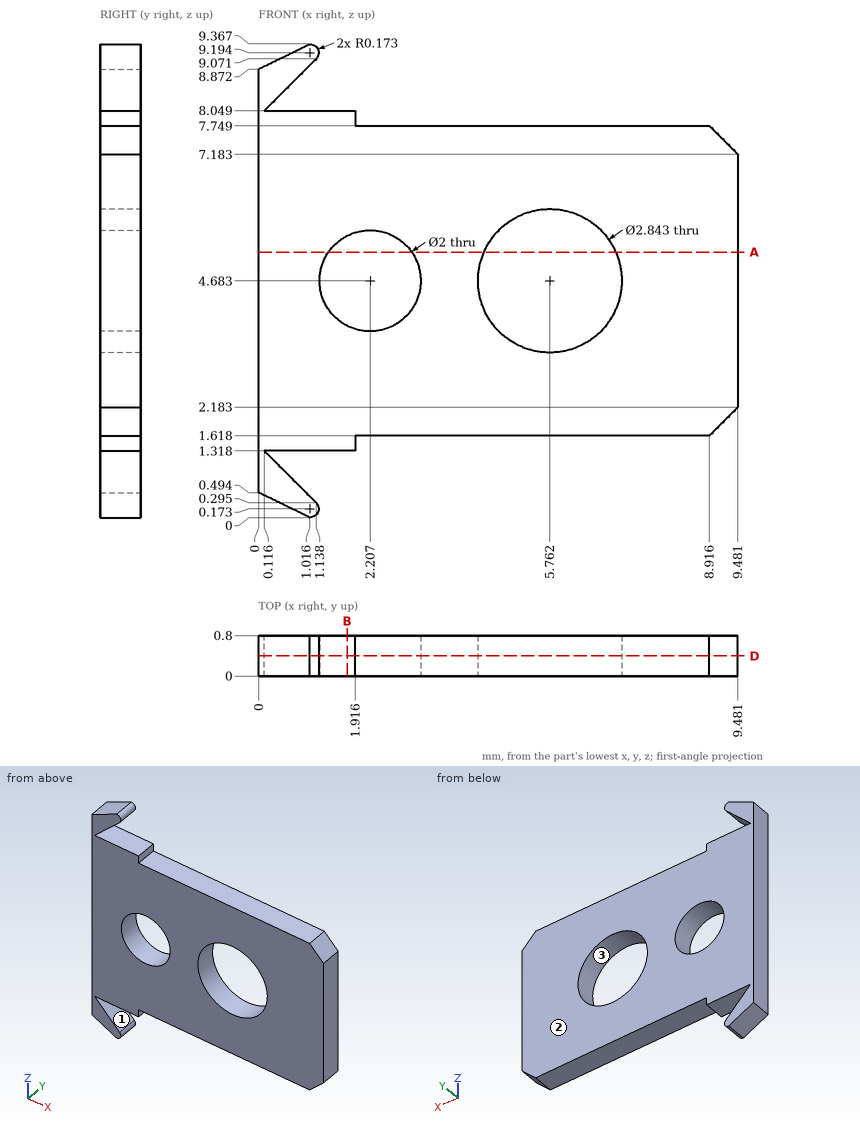
Answer from the drawing. Dimensions are ordinates in mm from the lowest x, y and z of the part. Round coordinates to 2 decimals unless told otherwise and drop trailing zeros. Write each loop counter-clockwise with the first axis right and the second up, starting at its lowest first coordinate (ties: lowest second). Pieces come first, ordered by that corner, then holes. Notation, with made-up numbers: M -21.5,-20.5 L -17.5,-20.5 A17 cw -17.5,8.5 Z; hole C 77.25,30.25 d11. An arc over 180 degrees is marked long. One line per item, written item: value.
Q1. Straight lines are drawn through the part: line 1 (X direction, y = 0.3, z = 4.75) (1 decimal); line 2 (X direction, y = 0.35, z = 4.5) (1 decimal); line 3 (Z direction, x = 8.5, y = 0.3). For each, find the intervals that lie inside material, in ascending order. Write a range as [from, to].
Data:
line 1: [0, 1.2], [3.2, 4.3], [7.2, 9.5]
line 2: [0, 1.2], [3.2, 4.4], [7.2, 9.5]
line 3: [1.62, 7.75]
Q2. A flat-ended cylindrical pin translates along its axis: pin 1 Ø2.5 at (x, z) = (5.76, 4.68) entering from +Y. Find the tip coordinate at first contact, or state that the pin passes through.
Data:
pin 1: through
Q3. Find section B-B on x = 1.75. Write down the section's boundary in (y, z).
Data:
outline: M 0,1.32 L 0.8,1.32 L 0.8,3.79 L 0,3.79 Z; M 0,5.57 L 0.8,5.57 L 0.8,8.05 L 0,8.05 Z
Q4. Find section A-A on z = 5.25. Write down the section's boundary in (x, y) (1 decimal).
Data:
outline: M 0,0 L 1.4,0 L 1.4,0.8 L 0,0.8 Z; M 3,0 L 4.5,0 L 4.5,0.8 L 3,0.8 Z; M 7.1,0 L 9.5,0 L 9.5,0.8 L 7.1,0.8 Z
Q5. For a pull along X with two mould halves and no side action, classify the marked faces 1, 2 and 3 as +X half, -X half, draft (parallel to the pull), parting line (faces both ways), or undercut.
Data:
face 1: +X half
face 2: draft
face 3: undercut
Q6. Find section D-D on y = 0.4. Count the separate pieces of the cut face and the enclosed holes in it.
Data:
separate pieces: 1
enclosed holes: 2
